Autodesk Fusion 360 part; units mm, degrees
sketch "Sketch1" plane through (0, 0, 0) normal (0, 0, 1) x (1, 0, 0)
  line L0 (25, -35) -> (-25, -35)
  line L1 (-25, -35) -> (-25, 35)
  line L2 (-25, 35) -> (25, 35)
  line L3 (25, 35) -> (25, -35)
  line L4 (25, -35) -> (-25, 35) construction
  line L5 (-25, -35) -> (25, 35) construction
  dimension "d1" = 50
  dimension "d2" = 70
extrude "Extrude1" add sketch "Sketch1" along normal blind 30
sketch "Sketch2" plane through (0, 35, 0) normal (0, 1, 0) x (-1, 0, 0)
  line L0 (-25, 0) -> (25, 0)
  line L1 (25, 0) -> (25, 30)
  line L2 (25, 30) -> (-25, 30)
  line L3 (-25, 30) -> (-25, 0)
sketch "Sketch3" plane through (0, -35, 0) normal (0, -1, 0) x (1, 0, 0)
  line L0 (-25, 0) -> (25, 0)
  line L1 (25, 0) -> (25, 30)
  line L2 (25, 30) -> (-25, 30)
  line L3 (-25, 30) -> (-25, 0)
  line L4 (-20.9844, 25.7659) -> (21.0156, 25.7659)
  line L5 (21.0156, 25.7659) -> (21.0156, 4.2659)
  line L6 (21.0156, 4.2659) -> (-20.9844, 4.2659)
  line L7 (-20.9844, 4.2659) -> (-20.9844, 25.7659)
  dimension "d5" = 42
  dimension "d6" = 21.5
extrude "Extrude2" cut sketch "Sketch3" against normal blind 65 contours L4 L5 L6 L7
Input: part model. Units: mm. Frame: model coordinates. A direction names the side the tool comes from. Give positions to 0.01 mm unless a question says otherwise; leave off trailing zeros. Order: outer loops, then holes, each group sorted by start corner. A loop starts at its lowest first (then second) coordinate and runs counter-clockwise, first axis right, second up.
1. Cut plane C-C (x = 18). Return loops of the section in (y, z).
Computed:
outline: (-35, 0) - (35, 0) - (35, 30) - (-35, 30) - (-35, 25.77) - (30, 25.77) - (30, 4.27) - (-35, 4.27) - close
2. Cut plane A-A (y = 16). Return loops of the section in (x, z), and give its area (3 significant figures).
Computed:
outline: (-25, 0) - (25, 0) - (25, 30) - (-25, 30) - close; hole (-20.98, 4.27) - (21.02, 4.27) - (21.02, 25.77) - (-20.98, 25.77) - close
area: 597 mm2
3. Line query: probe 1 along X at (y, z) = (29.5, 23); probe 2 along Z at (x, y) = (11, 20.5); probe 3 along Y at (x, z) = (2, 17.5). Output: solid intervals per line, ascending.
Computed:
probe 1: x = -25 to -20.98, 21.02 to 25
probe 2: z = 0 to 4.27, 25.77 to 30
probe 3: y = 30 to 35
4. Cut plane B-B (z = 5). Return loops of the section in (x, y), and give its area (3 significant figures).
Computed:
outline: (-25, -35) - (-20.98, -35) - (-20.98, 30) - (21.02, 30) - (21.02, -35) - (25, -35) - (25, 35) - (-25, 35) - close
area: 770 mm2
5. Pin query (flat end, axial travel): pin 1 Ø11 at (x, z) = (1.5, 10) entering from -Y. Return the tip coordinate at first contact, or that it passes through.
Computed:
pin 1: stops at y = 30
6. Draft query along Z for faces 3 (the face through (-20.984, -3, 15)), 4 (the face through (0, 0, 30)), 5 (the face through (0, 0, 0)), 6 (the face through (0, 35, 15)). Return one class per face: released by +Z, released by -Z, zero draft, split by the parting line, or undercut.
Computed:
face 3: undercut
face 4: released by +Z
face 5: released by -Z
face 6: zero draft
7. Set-up query: faces 1 (the face through (0, -35, 1)), 2 (the face through (0, 30, 15)). Return all of +Z, -Z, +X, -X, +Y, -Y with unobstructed straight access to the full face (end or side cutting, diameter ignored); none if empty.
Computed:
face 1: +Z, -Z, +X, -X, -Y
face 2: -Y
